Autodesk Inventor part; units mm, degrees
ref_plane "YZ Plane" through (0, 0, 0) normal (1, 0, 0) x (0, 1, 0)
ref_plane "XZ Plane" through (0, 0, 0) normal (0, 1, 0) x (-1, 0, 0)
ref_plane "XY Plane" through (0, 0, 0) normal (0, 0, 1) x (1, 0, 0)
sketch "Sketch1" plane through (0, 0, 0) normal (0, 0, 1) x (1, 0, 0)
  line L0 (0, 0) -> (-17.3205, 10) construction
  line L1 (5, -7.5) -> (-5, -7.5) construction
  line L2 (-5, -7.5) -> (-5, 7.5) construction
  line L3 (-5, 7.5) -> (5, 7.5) construction
  line L4 (5, 7.5) -> (5, -7.5) construction
  line L5 (5, -7.5) -> (-5, 7.5) construction
  line L6 (-5, -7.5) -> (5, 7.5) construction
  line L7 (-16.8753, 13.9751) -> (5.4452, 11.4751)
  arc A0 (9, 7.5) -> (5.4452, 11.4751) centre (5, 7.5) ccw
  line L8 (9, 7.5) -> (9, -7.5)
  arc A1 (5, -11.5) -> (9, -7.5) centre (5, -7.5) ccw
  line L9 (5, -11.5) -> (-5, -11.5)
  arc A2 (-8.2707, -9.8027) -> (-5, -11.5) centre (-5, -7.5) ccw
  line L10 (-8.2707, -9.8027) -> (-20.5912, 7.6973)
  arc A3 (-16.8753, 13.9751) -> (-20.5912, 7.6973) centre (-17.3205, 10) ccw
  dimension "d0" = 10
  dimension "d1" = 15
  dimension "d2" = 20
  dimension "d3" = 30
  dimension "d4" = 4
extrude "Extrusion1" add sketch "Sketch1" against normal blind 3
hole "Hole1" at (-17.3205, 10, 0) at (-5, 7.5, 0) at (5, 7.5, 0) at (5, -7.5, 0) at (-5, -7.5, 0) direction (0, 0, -1) diameter 3 depth 8 tip angle 118
hole "Hole2" at (0, 0, 0) direction (0, 0, -1) diameter 3 depth 8 tip angle 118
properties part number "LegBase_back"
Here's how the part is built. I have some questions about the finished solid (model axes, mm). Coordinates: 2 decimals unless noted, no trailing zeros. Order: outer loops, then holes, each group sorted by start corner. A loop starts at its lowest first (then second) coordinate and runs counter-clockwise, first axis right, second up.
Item 1: If we section it at C-C on y = 0: List the corners of the cut face in (x, z) for me, plus the area to 3 significant figures.
Result sheet:
outline: (-15.17, -3) - (-1.5, -3) - (-1.5, 0) - (-15.17, 0) - close; (1.5, -3) - (9, -3) - (9, 0) - (1.5, 0) - close
area: 63.5 mm2
Item 2: If we section it at B-B on z = -0.45: List the corners of the cut face in (x, y) for me.
Result sheet:
outline: (-20.59, 7.7) - (-8.27, -9.8) arc R4 ccw to (-5, -11.5) - (5, -11.5) arc R4 ccw to (9, -7.5) - (9, 7.5) arc R4 ccw to (5.45, 11.48) - (-16.88, 13.98) arc R4 ccw to start; hole circle Ø3 at (-17.32, 10); hole circle Ø3 at (-5, -7.5); hole circle Ø3 at (-5, 7.5); hole circle Ø3 at (0, 0); hole circle Ø3 at (5, -7.5); hole circle Ø3 at (5, 7.5)
Item 3: I need wall thicknesses on line 1 (Y direction, x = -5, z = -1.05); line 2 (X direction, y = 6.25, z = -1.8); line 3 (X direction, y = -7.5, z = -1.75). Which ranges of each line are inside material? Lowest first, please.
Result sheet:
line 1: y = -11.5 to -9, -6 to 6, 9 to 12.65
line 2: x = -19.57 to -5.83, -4.17 to 4.17, 5.83 to 9
line 3: x = -9.89 to -6.5, -3.5 to 3.5, 6.5 to 9
Item 4: For P1, Ø1, axis at x = -1, z = -1.5, coming from the +Y side; P2, Ø2.5, axis at x = -5, y = 7.5, coming from the +Z side, each with a flat end and sliding along its axis, tell me the tip position at first contact or that it passes through.
Result sheet:
P1: stops at y = 12.25
P2: passes through
Item 5: If we section it at D-D on y = -5: List the corners of the cut face in (x, z) for me.
Result sheet:
outline: (-11.65, -3) - (9, -3) - (9, 0) - (-11.65, 0) - close
Item 6: If we section it at A-A on x = 0: List the corners of the cut face in (y, z) for me, plus the area to 3 significant figures.
Result sheet:
outline: (-11.5, -3) - (-1.5, -3) - (-1.5, 0) - (-11.5, 0) - close; (1.5, -3) - (12.08, -3) - (12.08, 0) - (1.5, 0) - close
area: 61.8 mm2
Item 7: If we mould it in two halves opening along X, with no side actions, what happens to faces 1 (the face through (-14.34, -1.18, -1.48)), 2 (the face through (-0.07, 1.5, -1.52)), 3 (the face through (7.797, -10.359, -1.479)), 4 (the face through (-18.33, 11.11, -1.52))? For each: +X half, -X half, draft (parallel to the pull), parting line (faces both ways), or undercut.
Result sheet:
face 1: -X half
face 2: undercut
face 3: +X half
face 4: undercut
